Source: CAD feature listing. Evaluate the final solid. Frame: model axes, mm. Round coordinates to 2 decimals unless told otherwise and drop trailing zeros. Loops run counter-clockwise (first coordinate to the right, second up) from the corner with the lowest first, then second, coordinate; pieces in that order, holes last. Notation, with made-up numbers: M 12.5,85.5 L 53.5,85.5 A27 cw 53.5,106.5 Z; hole C 58,45 d9. An arc over 180 degrees is marked long. One line per item, written item: value.
from build123d import *

# Parameters (mm, degrees)
F1_DEPTH = 10
F2_R     = 10


with BuildPart() as f1:
    # F0 (on Top) → F1 (new body)
    with BuildSketch(Plane.XY):
        with BuildLine():
            ThreePointArc((0, 10), (2.928932, 2.928932), (10, 0))
            Line((10, 0), (40, 0))
            ThreePointArc((40, 0), (60, 20), (80, 0))
            Line((80, 0), (120, 0))
            Line((120, 0), (120, 120))
            Line((120, 120), (80, 120))
            ThreePointArc((80, 120), (60, 100), (40, 120))
            Line((40, 120), (0, 120))
            Line((0, 120), (0, 10))
        make_face()
    extrude(amount=F1_DEPTH)

    # F2
    f2_edges = [f1.edges().sort_by_distance(p)[0] for p in [
        (120, 120, 5),
    ]]
    fillet(f2_edges, radius=F2_R)


solid = f1.part
1. Ray query, line 1 (Y direction, x = 60, z = 6.75); line 2 (X direction, y = 103.5, z = 1.5); line 3 (X direction, y = 110, z = 7.75). Return the intervals inside material, ascending. Write a range as [from, to].
Report:
line 1: y = [20, 100]
line 2: x = [0, 48.7], [71.3, 120]
line 3: x = [0, 42.68], [77.32, 120]
2. Section query B-B (x = 60). Return the cut outline in (y, z).
Report:
outline: M 20,0 L 100,0 L 100,10 L 20,10 Z
3. Pull-direction query (X, two-part tool) for faces 1 (the face through (2.85, 3.01, 4.93)), 2 (the face through (100, 0, 5)), 3 (the face through (60, 100, 5)); classes: released by +X, released by -X, zero draft, split by the parting line, or undercut.
Report:
face 1: released by -X
face 2: zero draft
face 3: undercut
4. Pin query (flat end, axial travel): pin 1 (5 mm diameter, centred on x = 68, z = 6, fed in from +Y); pin 2 (5 mm diameter, centred on x = 64, z = 2, fed in from -Y); pin 3 (2 mm diameter, centred on x = 106.5, y = 13, fed in from -Z). Return the tip coordinate at first contact, or that it passes through.
Report:
pin 1: stops at y = 102.98
pin 2: stops at y = 18.91
pin 3: stops at z = 0
5. Section query A-A (z = 8). Return the cut outline in (x, y).
Report:
outline: M 0,10 A10 ccw 10,0 L 40,0 A20 cw 80,0 L 120,0 L 120,110 A10 ccw 110,120 L 80,120 A20 cw 40,120 L 0,120 Z
